```python
from build123d import *

# Parameters (mm, degrees)
SKETCH_2_W           = 26
SKETCH_2_H           = 6.5
EXTRUDE_1_DEPTH      = 20
SKETCH_3_W           = 19
SKETCH_3_H           = 14
CUT_EXTRUDE_2_DEPTH  = 25.72347063
EXTRUDE_3_DEPTH      = 0.5
EXTRUDE_3_DEPTH_BACK = 2
SKETCH_4_W           = 17
SKETCH_4_H           = 18.8
SKETCH_5_W           = 0.5
SKETCH_5_H           = 2
CUT_EXTRUDE_4_DEPTH  = 31.831963934
EXTRUDE_7_DEPTH      = 0.5
EXTRUDE_7_DEPTH_BACK = 6.5
SKETCH_6_W           = 26
SKETCH_6_H           = 18.8
CUT_EXTRUDE_8_DEPTH  = 35.122719704


with BuildPart() as part:
    # Эскиз2 → Вытянуть1 (new body)
    with BuildSketch(Plane(origin=(0, 0, 0), x_dir=(1, 0, 0), z_dir=(0, 1, 0))):
        Rectangle(SKETCH_2_W, SKETCH_2_H)
    extrude(amount=EXTRUDE_1_DEPTH)

    # Эскиз3 → Вытянуть2 (cut, through all)
    with BuildSketch(Plane.XY.offset(3.25)):
        with Locations((0, 10)):
            Rectangle(SKETCH_3_W, SKETCH_3_H)
    extrude(amount=-CUT_EXTRUDE_2_DEPTH, mode=Mode.SUBTRACT)

    # Эскиз4 → Вытянуть3 (add, two sides: drawn at the far end of the back side and taken through both)
    with BuildSketch(Plane.XZ.offset(-17).offset(-EXTRUDE_3_DEPTH_BACK)):
        Rectangle(SKETCH_4_W, SKETCH_4_H)
    extrude(amount=EXTRUDE_3_DEPTH + EXTRUDE_3_DEPTH_BACK)

    # Эскиз5 → Вытянуть4 (cut, through all)
    with BuildSketch(Plane(origin=(8.5, 0, 0), x_dir=(0, 0, -1), z_dir=(1, 0, 0))):
        with Locations((-3.5, 18)):
            Rectangle(SKETCH_5_W, SKETCH_5_H)
        with Locations((3.5, 18)):
            Rectangle(SKETCH_5_W, SKETCH_5_H)
    extrude(amount=-CUT_EXTRUDE_4_DEPTH, mode=Mode.SUBTRACT)

    # Эскиз6 → Вытянуть7 (add, two sides: drawn at the far end of the back side and taken through both)
    with BuildSketch(Plane(origin=(0, 3, 0), x_dir=(-1, 0, 0), z_dir=(0, 1, 0)).offset(-EXTRUDE_7_DEPTH_BACK)):
        Rectangle(SKETCH_6_W, SKETCH_6_H)
    extrude(amount=EXTRUDE_7_DEPTH + EXTRUDE_7_DEPTH_BACK)

    # Эскиз9 → Вытянуть8 (cut, through all)
    with BuildSketch(Plane(origin=(13, 0, 0), x_dir=(0, 0, -1), z_dir=(1, 0, 0))):
        Polygon((-3.25, 0), (-3.25, 3), (-3.75, 3), (-3.75, -3.5), (3.75, -3.5), (3.75, 3), (3.25, 3), (3.25, 0), align=None)
    extrude(amount=-CUT_EXTRUDE_8_DEPTH, mode=Mode.SUBTRACT)


solid = part.part
```
Geometry check sheet. Reference: the model listing, model coordinates, mm. A direction names the side the tool comes from. Coordinates: 2 decimals unless noted, no trailing zeros. Order: outer loops, then holes, each group sorted by start corner. A loop starts at its lowest first (then second) coordinate and runs counter-clockwise, first axis right, second up. Notation, with made-up numbers: (87, 71.5) - (96, 71.5) arc R14 ccw to (96, 88.5) - close; hole circle Ø8 at (76.5, 36.5). An arc over 180 degrees is marked (long way). Use one line per item in the form item = value.
1. Access from +Z, -Z, +X, -X, +Y, -Y to the whole of each face (thin tool, end or side, straight path). Record for faces 4 (the face through (0, 0, -3.75)), 5 (the face through (0, -3.5, 7)), 6 (the face through (0, 19, -7)), 7 (the face through (9, 17, 0)).
Here are the results:
face_4 = +X, -X, -Y
face_5 = +Z, -Z, +X, -X, -Y
face_6 = -Z, +X, -X, +Y
face_7 = +Z, -Z
2. Section check B-B (x = 3.25). Record the boundary of the cut face in (y, z).
Here are the results:
outline = (-3.5, -9.4) - (3.5, -9.4) - (3.5, 9.4) - (-3.5, 9.4) - (-3.5, 3.75) - (3, 3.75) - (3, 3.25) - (0, 3.25) - (0, -3.25) - (3, -3.25) - (3, -3.75) - (-3.5, -3.75) - close; (16.5, -9.4) - (19, -9.4) - (19, -3.75) - (17, -3.75) - (17, -3.25) - (20, -3.25) - (20, 3.25) - (17, 3.25) - (17, 3.75) - (19, 3.75) - (19, 9.4) - (16.5, 9.4) - close
3. Section check C-C (y = -0.75). Record the boundary of the cut face in (x, z).
Here are the results:
outline = (-13, -9.4) - (13, -9.4) - (13, -3.75) - (-13, -3.75) - close; (-13, 3.75) - (13, 3.75) - (13, 9.4) - (-13, 9.4) - close
4. Section check D-D (z = 5.5). Record the boundary of the cut face in (x, y).
Here are the results:
outline = (-13, -3.5) - (13, -3.5) - (13, 3.5) - (-13, 3.5) - close; (-8.5, 16.5) - (8.5, 16.5) - (8.5, 19) - (-8.5, 19) - close
5. Draft check along Y on faces 1 (the face through (0, 1, 3.25)), 2 (the face through (0, 16.5, 0)), 3 (the face through (0, 19, 7)). Enter one of: pulls with the +Y half, pulls with the -Y half, needs draft (parallel to the pull), parting line crosses it, or undercut.
Here are the results:
face_1 = needs draft
face_2 = undercut
face_3 = pulls with the +Y half
6. Gauge pin test, flat ends, axial feed: pin 1 (5 mm diameter, centred on x = 10, y = 14, fed in from -Z); pin 2 (5 mm diameter, centred on x = 0.5, y = 12.5, fed in from +Z). Record the tip position at first contact, or that the pin passes through.
Here are the results:
pin_1 = -3.25
pin_2 = through
7. Section check A-A (z = 2.5). Record the boundary of the cut face in (x, y), then the cut area to 3 significant figures.
Here are the results:
outline = (-13, 0) - (13, 0) - (13, 20) - (-13, 20) - close; hole (-9.5, 3.5) - (9.5, 3.5) - (9.5, 17) - (8.5, 17) - (8.5, 16.5) - (-8.5, 16.5) - (-8.5, 17) - (-9.5, 17) - close
area = 272 mm²
8. Scan lines: line 1 (Z direction, x = -8.5, y = 0.5); line 2 (X direction, y = 16, z = 1); line 3 (Y direction, x = -1.75, z = -0.25). Record each from-to range of solid material in increasing order.
Here are the results:
line_1 = -9.4 to -3.75, -3.25 to 3.25, 3.75 to 9.4
line_2 = -13 to -9.5, 9.5 to 13
line_3 = 0 to 3.5, 16.5 to 20
